```python
from build123d import *

# Parameters (mm, degrees)
F1_DEPTH = 100
F2_R     = 20


with BuildPart() as f1:
    # F0 (on Top) → F1 (new body)
    with BuildSketch(Plane.XY):
        Polygon((65.410733, -64.802073), (80.699533, 81.911258), (-68.142453, -58.360403), (-74.977696, -64.802073), align=None)
    extrude(amount=F1_DEPTH)

    # F2
    f2_edges = [f1.edges().sort_by_distance(p)[0] for p in [
        (73.055133, 8.554593, 100),
        (2.860919, 8.554593, 100),
        (-4.783481, -64.802073, 100),
        (65.410733, -64.802073, 50),
        (80.699533, 81.911258, 50),
        (73.055133, 8.554593, 0),
        (-74.977696, -64.802073, 50),
        (-4.783481, -64.802073, 0),
        (2.860919, 8.554593, 0),
    ]]
    fillet(f2_edges, radius=F2_R)


solid = f1.part
```
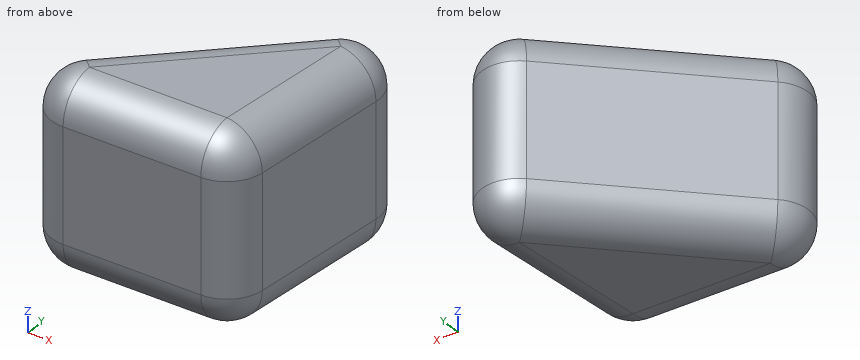
Check sheet for the modelled part. Datum: model origin and axes. Units: mm. Round coordinates to 2 decimals unless told otherwise and drop trailing zeros. Write each loop counter-clockwise with the first axis right and the second up, starting at its lowest first coordinate (ties: lowest second). Pieces come first, ordered by that corner, then holes. Notation, with made-up numbers: (-32.75, 58) -> (13.25, 58) arc R13 ccw to (13.25, 63) -> close; hole circle Ø6 at (4, 57). An arc over 180 degrees is marked (long way). One line per question, with ' | ' between items. Start each with the question number.
1. Scan lines: line 1 along X through (y, z) = (-35, 73); line 2 along Y through (x, z) = (48.5, 21); line 3 along X through (y, z) = (-18, 9.5). Record each from-to range of solid material in increasing order. Write a range as from..to.
2. Depth check by flat-ended pin: pin 1 (3 mm diameter, centred on x = 56, z = 79.5, fed in from -Y); pin 2 (6 mm diameter, centred on x = -27.5, z = 57, fed in from +Y); pin 3 (5 mm diameter, centred on x = 48.5, z = 17.5, fed in from -Y). Enter the tip coordinate at first touch or a pass-through.
3. Sectioned sample at A-A, the plane z = 87. Record the cut outline in (x, y) (3 decimals).
Taken from the geometry:
1) line 1: x = -42.03..68.52 | line 2: y = -64.77..49.26 | line 3: x = -20.97..67.29
2) pin 1: stops at y = -63.49 | pin 2: stops at y = -17.23 | pin 3: stops at y = -64.8
3) outline: (-37.444, -31.168) arc R18.735 ccw to (-24.595, -63.537) -> (47.387, -63.537) arc R18.735 ccw to (66.021, -46.744) -> (73.86, 28.48) arc R18.735 ccw to (42.376, 44.056) -> close
